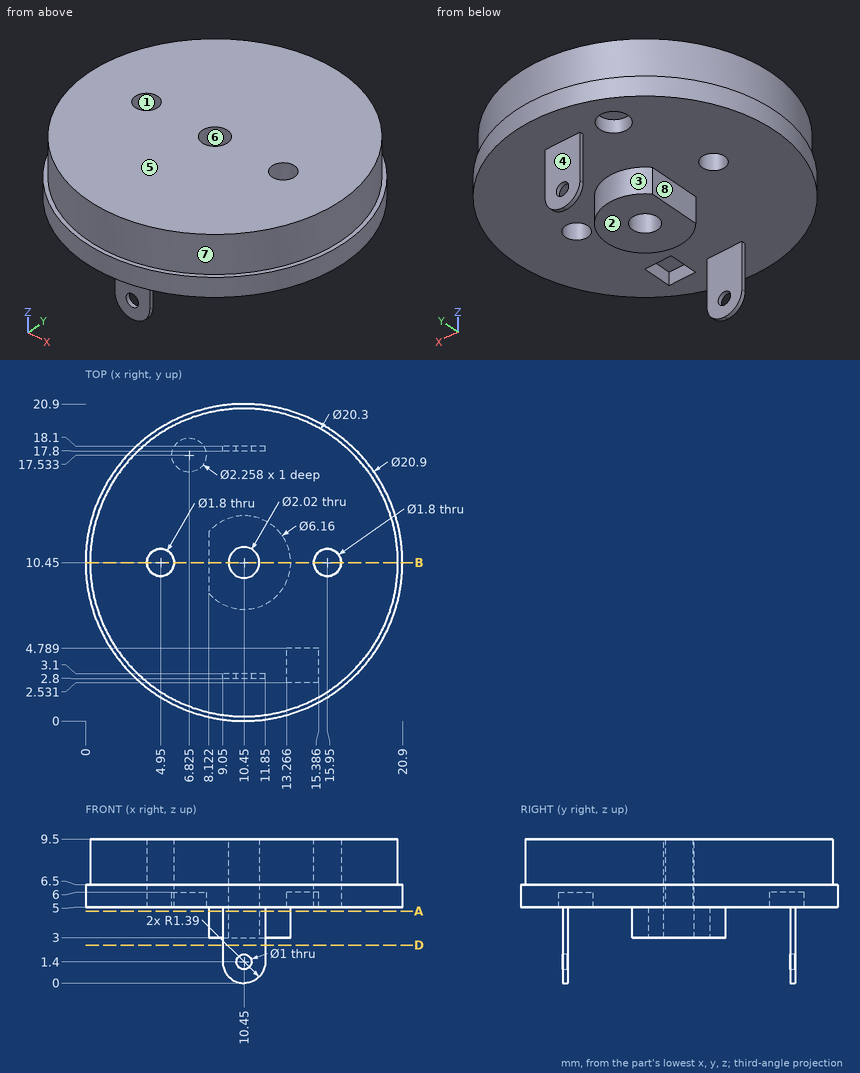
Check sheet for the drawn part. Datum: minimum x, y, z corner. Units: mm. A direction names the side the tool comes from. Round coordinates to 2 decimals unless told otherwise and drop trailing zeros. Write each loop counter-clockwise with the first axis right and the second up, starting at its lowest first coordinate (ties: lowest second). Pieces come first, ordered by that corner, then holes. Notation, with made-up numbers: (-3, -1) - (44, -1) arc R22 ccw to (44, 22) - close; hole circle Ø7 at (26, 27.5). An arc over 180 degrees is marked (long way). Return JSON: item names as keys, results as strings.
Q1. Cross-section at B-B (y = 10.45). Record the boundary of the cut face in (x, z).
Returned:
{"outline": "(0, 5) - (4.05, 5) - (4.05, 9.5) - (0.3, 9.5) - (0.3, 6.5) - (0, 6.5) - close; (5.85, 5) - (8.12, 5) - (8.12, 3) - (9.44, 3) - (9.44, 9.5) - (5.85, 9.5) - close; (11.46, 3) - (13.53, 3) - (13.53, 5) - (15.05, 5) - (15.05, 9.5) - (11.46, 9.5) - close; (16.85, 5) - (20.9, 5) - (20.9, 6.5) - (20.6, 6.5) - (20.6, 9.5) - (16.85, 9.5) - close"}
Q2. Cross-section at A-A (z = 4.75). Record the boundary of the cut face in (x, y).
Returned:
{"outline": "(8.12, 8.43) arc R3.08 ccw (long way) to (8.12, 12.47) - close; (9.05, 2.8) - (11.85, 2.8) - (11.85, 3.1) - (9.05, 3.1) - close; (9.05, 17.8) - (11.85, 17.8) - (11.85, 18.1) - (9.05, 18.1) - close; hole circle Ø2.02 at (10.45, 10.45)"}
Q3. Draft check along Y on the marked faces 6, 7 and 8. Enter one of: released by +Y, released by -Y, zero draft, split by the parting line, or undercut.
Returned:
{"face 6": "undercut", "face 7": "split by the parting line", "face 8": "zero draft"}
Q4. Cross-section at D-D (z = 2.5). Record the boundary of the cut face in (x, y).
Returned:
{"outline": "(9.05, 2.8) - (11.85, 2.8) - (11.85, 3.1) - (9.05, 3.1) - close; (9.05, 17.8) - (11.85, 17.8) - (11.85, 18.1) - (9.05, 18.1) - close"}
Q5. Scan lines: L1, parallel to X at y = 2.9, z = 1.4; L2, parallel to Z at x = 15, y = 17.25; L3, parallel to Y at x = 5.5, z = 8.5. Record each from-to range of solid material in increasing order. Write a range as from..to.
Returned:
{"L1": "x = 9.05..9.95, 10.95..11.85", "L2": "z = 5..9.5", "L3": "y = 1.59..9.74, 11.16..19.31"}
Q6. Depth check by flat-ended pin: P1, Ø0.7, axis at x = 6.5, y = 17, coming from the -Z side; P2, Ø5, axis at x = 17.5, y = 13, coming from the -Z side; P3, Ø0.8, axis at x = 10, z = 1.5, coming from the +Y side. Enter the tip coordinate at first touch or a pass-through.
Returned:
{"P1": "stops at z = 6", "P2": "stops at z = 5", "P3": "stops at y = 18.1"}
Q7. Access from +Z, -Z, +X, -X, +Y, -Y to the whole of each face (thin tool, end or side, straight path). Record for the marked faces 1, 2, 3, 4 and 5.
Returned:
{"face 1": "+Z, -Z", "face 2": "-Z, +X, -X", "face 3": "-Z", "face 4": "-Z, +X, -X, +Y", "face 5": "+Z, +X, -X, +Y, -Y"}
